For this review, take the finished solid that the model builds, in its own axes (mm). A direction names the side the tool comes from. Give positions to 0.01 mm unless a question says otherwise; leave off trailing zeros. Loops run counter-clockwise (first coordinate to the right, second up) from the corner with the lowest first, then second, coordinate; pieces in that order, holes last. Notation, with made-up numbers: (-7, 67) -> (20, 67) arc R31 ccw to (20, 105) -> close; hole circle Ø10 at (52, 23.5). An arc over 180 degrees is marked (long way). One line per question, with ' | ' between items. Start each with the question number.
(1) Insertion check: P1, Ø1.5, axis at x = -13.5, y = 0, coming from the +Z side; P2, Ø17, axis at x = 0, y = 0, coming from the +Z side. Each pin has a flat end and moves straight along its axis. Give the tip position at first contact, or say it passes through.
(2) Consider section A-A (y = 0). Write out the cut boundary in (x, z), and give its area (3 significant figures).
(3) Wall thickness on probe 1 along Y at (x, z) = (0, 5.6); probe 2 along X at (y, z) = (-2, 7.5); probe 3 along X at (y, z) = (1, 6): over which ranges is each line inside the solid? List them lowest first.
(4) Tool access review of faces 1 (the cylindrical face through (9.139, 14.334, 5.479)), 2 (the flat face through (0, -22.5, 5)): name each direction out of +Z, -Z, +X, -X, +Y, -Y from which nothing blocks a thin tool from reaching the whole face with its end or side.
(5) Consider section C-C (x = -18). Write out the cut boundary in (y, z), and give its area (3 significant figures).
from build123d import *

# Parameters (mm, degrees)
SKETCH1_W           = 45
SKETCH1_H           = 45
BOSS_EXTRUDE1_DEPTH = 10
SKETCH2_W           = 41
SKETCH2_H           = 41
CUT_EXTRUDE1_DEPTH  = 6
SKETCH3_R           = 17
SKETCH3_R_2         = 14
BOSS_EXTRUDE2_DEPTH = 3
FILLET2_R           = 3


with BuildPart() as part:
    # Sketch1 → Boss-Extrude1 (new body)
    with BuildSketch(Plane.XY):
        Rectangle(SKETCH1_W, SKETCH1_H)
    extrude(amount=BOSS_EXTRUDE1_DEPTH)

    # Sketch2 → Cut-Extrude1 (cut)
    with BuildSketch(Plane.XY.offset(10)):
        Rectangle(SKETCH2_W, SKETCH2_H)
    extrude(amount=-CUT_EXTRUDE1_DEPTH, mode=Mode.SUBTRACT)

    # Sketch3 → Boss-Extrude2 (add)
    with BuildSketch(Plane.XY.offset(4)):
        Circle(SKETCH3_R)
        Circle(SKETCH3_R_2, mode=Mode.SUBTRACT)
    extrude(amount=BOSS_EXTRUDE2_DEPTH)

    # Fillet2
    fillet2_edges = [part.edges().sort_by_distance(p)[0] for p in [
        (-22.5, 22.5, 5),
        (22.5, 22.5, 5),
        (22.5, -22.5, 5),
        (-22.5, -22.5, 5),
    ]]
    fillet(fillet2_edges, radius=FILLET2_R)


solid = part.part
A:
1) P1: stops at z = 7 | P2: stops at z = 4
2) outline: (-22.5, 0) -> (22.5, 0) -> (22.5, 10) -> (20.5, 10) -> (20.5, 4) -> (17, 4) -> (17, 7) -> (14, 7) -> (14, 4) -> (-14, 4) -> (-14, 7) -> (-17, 7) -> (-17, 4) -> (-20.5, 4) -> (-20.5, 10) -> (-22.5, 10) -> close | area: 222 mm^2
3) probe 1: y = -22.5 to -20.5, -17 to -14, 14 to 17, 20.5 to 22.5 | probe 2: x = -22.5 to -20.5, 20.5 to 22.5 | probe 3: x = -22.5 to -20.5, -16.97 to -13.96, 13.96 to 16.97, 20.5 to 22.5
4) face 1: +Z | face 2: +Z, -Z, +X, -X, -Y
5) outline: (-22.5, 0) -> (22.5, 0) -> (22.5, 10) -> (20.5, 10) -> (20.5, 4) -> (-20.5, 4) -> (-20.5, 10) -> (-22.5, 10) -> close | area: 204 mm^2
